from build123d import *

# Parameters (mm, degrees)
INSERT_SKETCH_R       = 5
INSERT_SKETCH_R_2     = 3.2
INSERT_DEPTH          = 15
SKETCH2_R             = 4.95
SKETCH2_R_2           = 3.2
CHUCK_SHOULDER_DEPTH  = 0.95
SKETCH4_R             = 3.75
SKETCH4_R_2           = 3.2
CHUCK_MINOR_DIA_DEPTH = 1
SKETCH5_R             = 4.95
SKETCH5_R_2           = 3.2
CHUCK_TOP_DEPTH       = 1.25
CHUCK_TOP_FILLET_R    = 0.5


with BuildPart() as part:
    # Insert Sketch → Insert (new body)
    with BuildSketch(Plane.XY):
        Circle(INSERT_SKETCH_R)
        Circle(INSERT_SKETCH_R_2, mode=Mode.SUBTRACT)
    extrude(amount=INSERT_DEPTH)

    # Sketch2 → chuck shoulder (add)
    with BuildSketch(Plane.XY.offset(15)):
        with Locations(Location((0, 0, 0), (0, 0, 180))):
            Circle(SKETCH2_R)
        Circle(SKETCH2_R_2, mode=Mode.SUBTRACT)
    extrude(amount=CHUCK_SHOULDER_DEPTH)

    # Sketch4 → chuck minor dia (add)
    with BuildSketch(Plane.XY.offset(15.95)):
        Circle(SKETCH4_R)
        Circle(SKETCH4_R_2, mode=Mode.SUBTRACT)
    extrude(amount=CHUCK_MINOR_DIA_DEPTH)

    # Sketch5 → chuck top (add)
    with BuildSketch(Plane.XY.offset(16.95)):
        with Locations(Location((0, 0, 0), (0, 0, 180))):
            Circle(SKETCH5_R)
        Circle(SKETCH5_R_2, mode=Mode.SUBTRACT)
    extrude(amount=CHUCK_TOP_DEPTH)

    # chuck top fillet
    chuck_top_fillet_edges = [part.edges().sort_by_distance(p)[0] for p in [
        (4.95, 0, 18.2),
    ]]
    fillet(chuck_top_fillet_edges, radius=CHUCK_TOP_FILLET_R)


solid = part.part
CAD build for the part. Positions are in the model's coordinates, mm. A direction names the side the tool comes from. Round coordinates to 2 decimals unless told otherwise and drop trailing zeros. Loops run counter-clockwise (first coordinate to the right, second up) from the corner with the lowest first, then second, coordinate; pieces in that order, holes last.
(1) Two-plate mould, pull along Z, no slides. Class faces 4 (the cylindrical face through (-2.539, -1.947, 8.973)), 5 (the flat face through (-3, 2, 18.2)), 6 (the cylindrical face through (-3.746, 0.165, 16.443)): +Z half, -Z half, draft (parallel to the pull), parting line (faces both ways), or undercut.
(2) Which spindle directions (+Z, -Z, +X, -X, +Y, -Y) get a long thin tool onto all of the face, cutting with end or side? Do faces 1 (the cylindrical face through (-4.72, -1.49, 17.32)), 2 (the flat face through (1, -4, 16.95)), 3 (the flat face through (1, -3.3, 0)). Say none if no direction does.
(3) Wall check: line 1 along Y through (x, z) = (0, 6.25); line 2 along Z through (x, y) = (4, 0.5); line 3 along Y through (x, z) = (-0.75, 7.75). Give the ranges that are in metal, low to high.
(4) Drop flat-ended pins along their axis: pin 1 (4 mm diameter, centred on x = 0, y = 0, fed in from -Z); pin 2 (6 mm diameter, centred on x = -3.5, z = 14, fed in from -Y); pin 3 (2 mm diameter, centred on y = -3.5, z = 3, fed in from +X). Give the stop position or say it passes through.
(5) Cut at C-C (z = 5). Give the cut face in (x, y).
(6) Cut at A-A (y = 0). Give the cut face in (x, z).
Findings below:
1. face 4: draft
1. face 5: +Z half
1. face 6: undercut
2. face 1: +Z
2. face 2: none
2. face 3: -Z, +X, -X, +Y, -Y
3. line 1: y = -5 to -3.2, 3.2 to 5
3. line 2: z = 0 to 15.95, 16.95 to 18.2
3. line 3: y = -4.94 to -3.11, 3.11 to 4.94
4. pin 1: passes through
4. pin 2: stops at y = -4.97
4. pin 3: stops at x = 4.33
5. outline: circle Ø10 at (0, 0); hole circle Ø6.4 at (0, 0)
6. outline: (-5, 0) - (-3.2, 0) - (-3.2, 18.2) - (-4.45, 18.2) arc R0.5 ccw to (-4.95, 17.7) - (-4.95, 16.95) - (-3.75, 16.95) - (-3.75, 15.95) - (-4.95, 15.95) - (-4.95, 15) - (-5, 15) - close; (3.2, 0) - (5, 0) - (5, 15) - (4.95, 15) - (4.95, 15.95) - (3.75, 15.95) - (3.75, 16.95) - (4.95, 16.95) - (4.95, 17.7) arc R0.5 ccw to (4.45, 18.2) - (3.2, 18.2) - close
